from build123d import *

# Parameters (mm, degrees)
DODANIE_WYCI_GNI_CIE1_DEPTH = 6
SZKIC3_R                    = 5.05
WYTNIJ_WYCI_GNI_CIE1_DEPTH  = 418.898779611
SZKIC4_OUTSIDE_W            = 37.616
SZKIC4_OUTSIDE_H            = 51.616
SZKIC4_OUTSIDE_R            = 12.5
WYTNIJ_WYCI_GNI_CIE2_DEPTH  = 10


with BuildPart() as part:
    # Szkic1 → Dodanie-wyciągnięcie1 (new body)
    with BuildSketch(Plane(origin=(0, -358.273993717, 0), x_dir=(1, 0, 0), z_dir=(0, 1, 0))):
        with BuildLine():
            Line((-393.068007623, -130.155243162), (-375.068007623, -130.155243162))
            ThreePointArc((-375.068007623, -130.155243162), (-372.239580498, -128.983670286), (-371.068007623, -126.155243162))
            Line((-371.068007623, -126.155243162), (-371.068007623, -94.155243162))
            ThreePointArc((-371.068007623, -94.155243162), (-372.239580498, -91.326816037), (-375.068007623, -90.155243162))
            Line((-375.068007623, -90.155243162), (-393.068007623, -90.155243162))
            ThreePointArc((-393.068007623, -90.155243162), (-395.896434748, -91.326816037), (-397.068007623, -94.155243162))
            Line((-397.068007623, -94.155243162), (-397.068007623, -126.155243162))
            ThreePointArc((-397.068007623, -126.155243162), (-395.896434748, -128.983670286), (-393.068007623, -130.155243162))
        make_face()
    extrude(amount=DODANIE_WYCI_GNI_CIE1_DEPTH)

    # Szkic3 → Wytnij-wyciągnięcie1 (cut, through all)
    with BuildSketch(Plane(origin=(0, -352.273993717, 0), x_dir=(1, 0, 0), z_dir=(0, 1, 0))):
        with Locations(Location((-384.068007623, -110.155243162, 0), (0, 0, 270))):
            Circle(SZKIC3_R)
    extrude(amount=-WYTNIJ_WYCI_GNI_CIE1_DEPTH, mode=Mode.SUBTRACT)

    # Szkic4 outside → Wytnij-wyciągnięcie2 (cut)
    with BuildSketch(Plane(origin=(0, -352.273993717, 0), x_dir=(1, 0, 0), z_dir=(0, 1, 0))):
        with Locations((-384.068, -110.155)):
            Rectangle(SZKIC4_OUTSIDE_W, SZKIC4_OUTSIDE_H)
        with Locations(Location((-384.068007623, -110.155243162, 0), (0, 0, 270))):
            Circle(SZKIC4_OUTSIDE_R, mode=Mode.SUBTRACT)
    extrude(amount=-WYTNIJ_WYCI_GNI_CIE2_DEPTH, mode=Mode.SUBTRACT)


solid = part.part
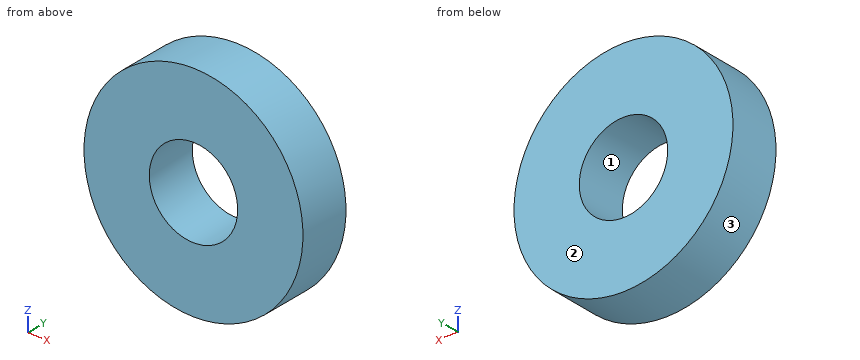
Work out the finished part from the listing and answer in its coordinate system (mm). Face numbers are marked on the shaded views. Coordinates: 2 decimals unless noted, no trailing zeros. Loops run counter-clockwise (first coordinate to the right, second up) from the corner with the lowest first, then second, coordinate; pieces in that order, holes last. Notation, with made-up numbers: (-20, 76.25) -> (32, 76.25) arc R18 cw to (32, 86.25) -> close; hole circle Ø11 at (-3.75, -2.5). An arc over 180 degrees is marked (long way). Write each question's results on one line, items separated by ' | '. Start each with the question number.
1) Consider line 1 along Z through (x, y) = (-384.25, -355.7); line 2 along Z through (x, y) = (-383, -355.1); line 3 along X through (y, z) = (-357, 113.5). Determine where each line is inside the solid, lowest interval first.
2) Find section B-B on z = 114.5. Determine the outline of the cut face in (x, y), then the cut area to 3 significant figures.
3) Find section D-D on z = 102. Determine the outline of the cut face in (x, y).
4) Find section C-C on y = -355.45. Determine the outline of the cut face in (x, z), then the cut area to 3 significant figures.
5) The mould has two halves that part along Z. Classify the marked faces 1, 2 and 3: pulls with the +Z half, pulls with the -Z half, needs draft (parallel to the pull), parting line crosses it, or undercut.
6) Flat-ended cylindrical pins translate along their axes: P1, Ø3, axis at x = -389.5, y = -354, coming from the -Z side; P2, Ø3, axis at x = -392, y = -357.5, coming from the -Z side; P3, Ø8, axis at x = -384.07, z = 110.16, coming from the -Y side. Find the tip coordinate at first contact, or state that the pin passes through.
7) Find section A-A on x = -384.5. Determine the outline of the cut face in (y, z), then the cut area to 3 significant figures.
Response values:
1) line 1: z = 97.66 to 105.11, 115.2 to 122.65 | line 2: z = 97.7 to 105.22, 115.09 to 122.61 | line 3: x = -396.11 to -387.85, -380.28 to -372.02
2) outline: (-395.79, -358.27) -> (-386.64, -358.27) -> (-386.64, -352.27) -> (-395.79, -352.27) -> close; (-381.49, -358.27) -> (-372.35, -358.27) -> (-372.35, -352.27) -> (-381.49, -352.27) -> close | area: 110 mm^2
3) outline: (-393.54, -358.27) -> (-374.59, -358.27) -> (-374.59, -352.27) -> (-393.54, -352.27) -> close
4) outline: circle Ø25 at (-384.07, 110.16); hole circle Ø10.1 at (-384.07, 110.16) | area: 411 mm^2
5) face 1: undercut | face 2: needs draft | face 3: parting line crosses it
6) P1: stops at z = 98.29 | P2: stops at z = 99.44 | P3: passes through
7) outline: (-358.27, 97.66) -> (-352.27, 97.66) -> (-352.27, 105.12) -> (-358.27, 105.12) -> close; (-358.27, 115.19) -> (-352.27, 115.19) -> (-352.27, 122.65) -> (-358.27, 122.65) -> close | area: 89.5 mm^2
